Design review of the part built by this model. Coordinates are the model's own, in mm. Face numbers are marked on the shaded views. Give positions to 0.01 mm unless a question says otherwise; leave off trailing zeros. Loops run counter-clockwise (first coordinate to the right, second up) from the corner with the lowest first, then second, coordinate; pieces in that order, holes last. Notation, with made-up numbers: (88.5, -16.5) - (127.5, -16.5) arc R14 cw to (127.5, -11.5) - close; hole circle Ø7 at (3, -22). An arc over 180 degrees is marked (long way). One line per item, written item: value. Start each with the question number.
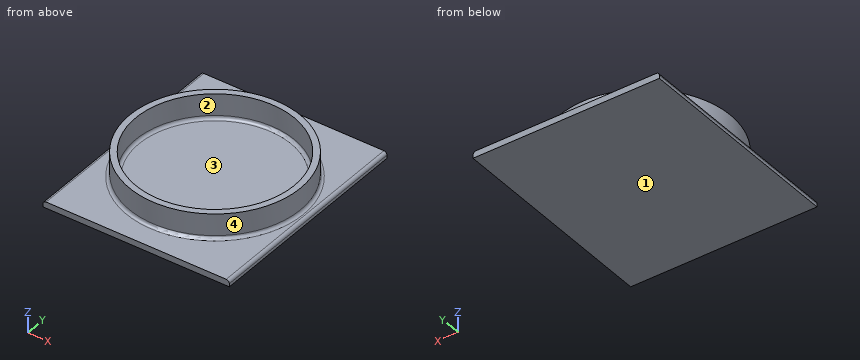
```python
from build123d import *

# Parameters (mm, degrees)
F0_W     = 76.2
F0_H     = 88.9
F1_DEPTH = 2.54
F2_R     = 34.925
F3_DEPTH = 10.16
F4_R     = 32.385
F5_DEPTH = 10.16
F6_R     = 1.27


with BuildPart() as f1:
    # F0 (on Top) → F1 (new body)
    with BuildSketch(Plane.XY):
        with Locations((38.1, 44.45)):
            Rectangle(F0_W, F0_H)
    extrude(amount=F1_DEPTH)

    # F2 (on face) → F3 (join)
    with BuildSketch(Plane.XY.offset(2.54)):
        with Locations((38.1, 44.45)):
            Circle(F2_R)
    extrude(amount=F3_DEPTH)

    # F4 (on face) → F5 (cut)
    with BuildSketch(Plane.XY.offset(12.7)):
        with Locations((38.1, 44.45)):
            Circle(F4_R)
    extrude(amount=-F5_DEPTH, mode=Mode.SUBTRACT)

    # F6
    f6_edges = [f1.edges().sort_by_distance(p)[0] for p in [
        (5.715, 44.45, 2.54),
        (0, 44.45, 2.54),
        (76.2, 44.45, 2.54),
        (3.175, 44.45, 2.54),
    ]]
    fillet(f6_edges, radius=F6_R)


solid = f1.part
```
(1) Take a section at B-B on z = 6. State the section outline as (x, y) points (3 decimals).
(2) Take a section at D-D on y = 82. State the section outline as (x, z) points.
(3) For pin 1 Ø1 at (y, z) = (52.5, 11) entering from +X; pin 2 Ø1 at (x, z) = (13, 6.5) entering from +Y; pin 3 Ø2 at (y, z) = (45, 11) entering from -X (3 decimals), all flat-tipped, find the tip position at first contact; note any pin that passes through.
(4) Take a section at C-C on y = 44.45. State the section outline as (x, z) points (3 decimals).
(5) To check wall thickness, follow L1, parallel to Y at x = 38.1, z = 9.5 (3 decimals); L2, parallel to X at y = 65, z = 10; L3, parallel to Z at x = 53, y = 45.5. State the ranges of each line that lie inside material, in increasing order. Write a range as from..to.
(6) Draft analysis for pull direction Y (two halves, no side actions). For the marked faces 1, 2, 3 and 4, state which applies: pulls with the +Y half, pulls with the -Y half, needs draft (parallel to the pull), parting line crosses it, or undercut.
(7) Take a section at A-A on x = 38.1. State the section outline as (y, z) points (3 decimals).
Here are the results:
1. outline: circle Ø69.85 at (38.1, 44.45); hole circle Ø64.77 at (38.1, 44.45)
2. outline: (0, 0) - (76.2, 0) - (76.2, 1.27) arc R1.27 ccw to (74.93, 2.54) - (1.27, 2.54) arc R1.27 ccw to (0, 1.27) - close
3. pin 1: x = 72.2
3. pin 2: y = 69.24
3. pin 3: x = 3.175
4. outline: (0, 0) - (76.2, 0) - (76.2, 1.27) arc R1.27 ccw to (74.93, 2.54) - (74.295, 2.54) arc R1.27 cw to (73.025, 3.81) - (73.025, 12.7) - (70.485, 12.7) - (70.485, 3.81) arc R1.27 cw to (69.215, 2.54) - (6.985, 2.54) arc R1.27 cw to (5.715, 3.81) - (5.715, 12.7) - (3.175, 12.7) - (3.175, 3.81) arc R1.27 cw to (1.905, 2.54) - (1.27, 2.54) arc R1.27 ccw to (0, 1.27) - close
5. L1: 9.525..12.065, 76.835..79.375
5. L2: 9.86..13.07, 63.13..66.34
5. L3: 0..2.54
6. face 1: needs draft
6. face 2: undercut
6. face 3: undercut
6. face 4: parting line crosses it
7. outline: (0, 0) - (88.9, 0) - (88.9, 2.54) - (80.645, 2.54) arc R1.27 cw to (79.375, 3.81) - (79.375, 12.7) - (76.835, 12.7) - (76.835, 3.81) arc R1.27 cw to (75.565, 2.54) - (13.335, 2.54) arc R1.27 cw to (12.065, 3.81) - (12.065, 12.7) - (9.525, 12.7) - (9.525, 3.81) arc R1.27 cw to (8.255, 2.54) - (0, 2.54) - close
